Input: part model. Units: mm. Frame: model coordinates. A direction names the side the tool comes from. Round coordinates to 2 decimals unless told otherwise and drop trailing zeros. Loops run counter-clockwise (first coordinate to the right, second up) from the corner with the lowest first, then second, coordinate; pieces in that order, holes last. Notation, with made-up numbers: (-3.75, -32) - (53.25, -32) arc R22 ccw to (53.25, -23) - close; hole circle Ø9 at (0, 24). An arc over 180 degrees is marked (long way). Use CSV: the item, a comma, the result in double quotes. Start each with the question number.
1. Material intervals for probe 1 along X at (y, z) = (0, 6.5); probe 2 along Z at (x, y) = (-2, 1); probe 3 along Y at (x, z) = (-27, 59), sorted ascending. Write a range as from..to.
2. Pull-direction query (Y, two-part tool) for faces 3 (the flat face through (24.7, 33.9, 33.5)), 4 (the flat face through (0, 0, 11)), 5 (the flat face through (-1, -2, 70)); classes: +Y half, -Y half, draft (parallel to the pull), parting line (faces both ways), or undercut.
3. Cut plane B-B (y = 0). Return loops of the section in (x, z), and give its area (3 significant figures).
4. Pin query (flat end, axial travel): P1, Ø12, axis at x = -30.5, z = 51.5, coming from the +Y side; P2, Ø3.5, axis at x = 1.5, y = 0, coming from the -Z side; P3, Ø5, axis at y = -2, z = 23, coming from the +X side. Return the tip coordinate at first contact, or that it passes through.
5. Access query for faces 1 (the cylindrical face through (3.233, 1.341, 5.423)), 2 (the flat face through (34.81, 11.02, 68.99)). Directions: +Z, -Z, +X, -X, +Y, -Y. A direction counts if a zero-diameter tool reaches every point of the face in a straight line with its end or side. Return the directions, or none.
6. Cut plane A-A (z = 14). Return loops of the section in (x, y).
7. Cut plane C-C (x = 18). Return loops of the section in (y, z), and give its area (3 significant figures).
8. Cut plane D-D (y = -15). Return loops of the section in (x, z), and give its area (3 significant figures).
Autodesk Fusion 360 part; units mm, degrees
sketch "Sketch1" plane through (0, 0, 0) normal (0, 0, 1) x (1, 0, 0)
  line L0 (-29.563, 30.3671) -> (-41.7663, -7.1908)
  line L1 (-38.0163, -18.7321) -> (-6.0676, -41.9442)
  line L2 (6.0676, -41.9442) -> (38.0163, -18.7321)
  line L3 (41.7663, -7.1908) -> (29.563, 30.3671)
  line L4 (19.7453, 37.5) -> (-19.7453, 37.5)
  line L5 (-29.563, 30.3671) -> (-19.7453, 37.5)
  line L6 (-41.7663, -7.1908) -> (-38.0163, -18.7321)
  line L7 (-6.0676, -41.9442) -> (6.0676, -41.9442)
  line L8 (38.0163, -18.7321) -> (41.7663, -7.1908)
  line L9 (29.563, 30.3671) -> (19.7453, 37.5)
  point P0 (-27.2453, 37.5)
  point P1 (-44.0839, -14.3237)
  point P2 (0, -46.3525)
  point P3 (44.0839, -14.3237)
  point P4 (27.2453, 37.5)
extrude "Extrude1" add sketch "Sketch1" along normal blind 70
sketch "Sketch2" plane through (0, 0, 0) normal (0, 0, -1) x (1, 0, 0)
  line L0 (-41.7663, 7.1908) -> (-29.563, -30.3671)
  line L1 (-29.563, -30.3671) -> (-19.7453, -37.5)
  line L2 (-19.7453, -37.5) -> (19.7453, -37.5)
  line L3 (19.7453, -37.5) -> (29.563, -30.3671)
  line L4 (29.563, -30.3671) -> (41.7663, 7.1908)
  line L5 (41.7663, 7.1908) -> (38.0163, 18.7321)
  line L6 (38.0163, 18.7321) -> (6.0676, 41.9442)
  line L7 (6.0676, 41.9442) -> (-6.0676, 41.9442)
  line L8 (-6.0676, 41.9442) -> (-38.0163, 18.7321)
  line L9 (-38.0163, 18.7321) -> (-41.7663, 7.1908)
  circle A0 centre (0, 0) radius 3.5
  dimension "d13" = 7
extrude "Extrude2" cut sketch "Sketch2" against normal blind 11 contours A0
chamfer "Chamfer1" distance 2 angle 45 1 faces at (-0.7952, -10.1031, 70)
Established:
1,probe 1,"x = -39.43..-3.5, 3.5..39.43"
1,probe 2,"z = 11..70"
1,probe 3,"y = -26.74..32.23"
2,face 3,"+Y half"
2,face 4,"undercut"
2,face 5,"draft"
3,outline,"(-39.43, 0) - (-3.5, 0) - (-3.5, 11) - (3.5, 11) - (3.5, 0) - (39.43, 0) - (39.43, 68) - (37.33, 70) - (-37.33, 70) - (-39.43, 68) - close"
3,area,"5,440 mm2"
4,P1,"stops at y = 34.05"
4,P2,"stops at z = 11"
4,P3,"stops at x = 40.89"
5,face 1,"-Z"
5,face 2,"+Z, +X, +Y"
6,outline,"(-41.77, -7.19) - (-38.02, -18.73) - (-6.07, -41.94) - (6.07, -41.94) - (38.02, -18.73) - (41.77, -7.19) - (29.56, 30.37) - (19.75, 37.5) - (-19.75, 37.5) - (-29.56, 30.37) - close"
7,outline,"(-33.27, 0) - (37.5, 0) - (37.5, 68) - (35.5, 70) - (-30.8, 70) - (-33.27, 68) - close"
7,area,"4,950 mm2"
8,outline,"(-39.23, 0) - (39.23, 0) - (39.23, 68) - (37.13, 70) - (-37.13, 70) - (-39.23, 68) - close"
8,area,"5,490 mm2"
